Verification items for the finished model (mm, model axes). A direction names the side the tool comes from. Coordinates: 2 decimals unless noted, no trailing zeros. Write each loop counter-clockwise with the first axis right and the second up, starting at its lowest first coordinate (ties: lowest second). Pieces come first, ordered by that corner, then holes. Notation, with made-up numbers: M 32.5,80.25 L 71.5,80.25 A18 cw 71.5,103.25 Z; hole C -10,69.25 d5. An arc over 180 degrees is marked long. Answer in a Markdown table with one row per item.
from build123d import *

# Parameters (mm, degrees)
SKETCH1_W           = 200
SKETCH1_H           = 50
BOSS_EXTRUDE2_DEPTH = 3.18
SKETCH3_W           = 3.18
SKETCH3_H           = 17.5
CUT_EXTRUDE1_DEPTH  = 104.12668132
SKETCH4_R           = 1.55
CUT_EXTRUDE2_DEPTH  = 104.12668132


with BuildPart() as part:
    # Sketch1 → Boss-Extrude2 (new body)
    with BuildSketch(Plane.XY):
        Rectangle(SKETCH1_W, SKETCH1_H)
    extrude(amount=BOSS_EXTRUDE2_DEPTH)

    # Sketch3 → Cut-Extrude1 (cut, through all)
    with BuildSketch(Plane.XY.offset(3.18)):
        with Locations((-98.41, 16.25)):
            Rectangle(SKETCH3_W, SKETCH3_H)
        with Locations((-98.41, -16.25)):
            Rectangle(SKETCH3_W, SKETCH3_H)
        with Locations((98.41, 16.25)):
            Rectangle(SKETCH3_W, SKETCH3_H)
        with Locations((98.41, -16.25)):
            Rectangle(SKETCH3_W, SKETCH3_H)
    extrude(amount=-CUT_EXTRUDE1_DEPTH, mode=Mode.SUBTRACT)

    # Sketch4 → Cut-Extrude2 (cut, through all)
    with BuildSketch(Plane.XY.offset(3.18)):
        with Locations((-98, -0.707640919)):
            Circle(SKETCH4_R)
        with Locations((98.002158409, -0.27875217)):
            Circle(SKETCH4_R)
    extrude(amount=-CUT_EXTRUDE2_DEPTH, mode=Mode.SUBTRACT)


solid = part.part
1) Thickness scan on L1, parallel to Y at x = -98, z = 2.15; L2, parallel to X at y = -22, z = 3; L3, parallel to X at y = 0, z = 2.3. Record the ranges inside material, lowest first. Write a range as [from, to].
Response values:
| item | result |
|---|---|
| L1 | y = [-7.5, -2.26], [0.84, 7.5] |
| L2 | x = [-96.82, 96.82] |
| L3 | x = [-100, -99.38], [-96.62, 96.48], [99.53, 100] |
2) Sectioned sample at A-A (z = 1.3). Record the cut outline in (x, y).
Response values:
| item | result |
|---|---|
| outline | M -100,-7.5 L -96.82,-7.5 L -96.82,-25 L 96.82,-25 L 96.82,-7.5 L 100,-7.5 L 100,7.5 L 96.82,7.5 L 96.82,25 L -96.82,25 L -96.82,7.5 L -100,7.5 Z; hole C -98,-0.71 d3.1; hole C 98,-0.28 d3.1 |
3) Release check for a two-part mould opening along X. For faces 5 (the face through (-96.522, -0.242, 1.612)), 6 (the face through (98, 7.5, 2)), 7 (the face through (-96.82, -16, 2)) record: +X half, -X half, draft (parallel to the pull), parting line (faces both ways), or undercut.
Response values:
| item | result |
|---|---|
| face 5 | undercut |
| face 6 | draft |
| face 7 | -X half |
4) Tool access check on faces 1 (the face through (-98, -7.5, 2)), 2 (the face through (96.82, 16, 2)), 3 (the face through (-96.82, 16, 2)), 4 (the face through (98, -7.5, 2)). Record the directions out of +Z, -Z, +X, -X, +Y, -Y that give a thin tool (end or side, any length) a straight path to the whole face; none if there is none.
Response values:
| item | result |
|---|---|
| face 1 | +Z, -Z, -X, -Y |
| face 2 | +Z, -Z, +X, +Y |
| face 3 | +Z, -Z, -X, +Y |
| face 4 | +Z, -Z, +X, -Y |
5) Sectioned sample at B-B (y = 18.5). Record the cut outline in (x, z).
Response values:
| item | result |
|---|---|
| outline | M -96.82,0 L 96.82,0 L 96.82,3.18 L -96.82,3.18 Z |
6) Depth check by flat-ended pin: pin 1 (1 mm diameter, centred on y = 12.5, z = 2, fed in from +X); pin 2 (1 mm diameter, centred on x = -98, z = 2, fed in from +Y); pin 3 (1 mm diameter, centred on x = 98.5, z = 2, fed in from -Y). Enter the tip coordinate at first touch or a pass-through.
Response values:
| item | result |
|---|---|
| pin 1 | stops at x = 96.82 |
| pin 2 | stops at y = 7.5 |
| pin 3 | stops at y = -7.5 |
